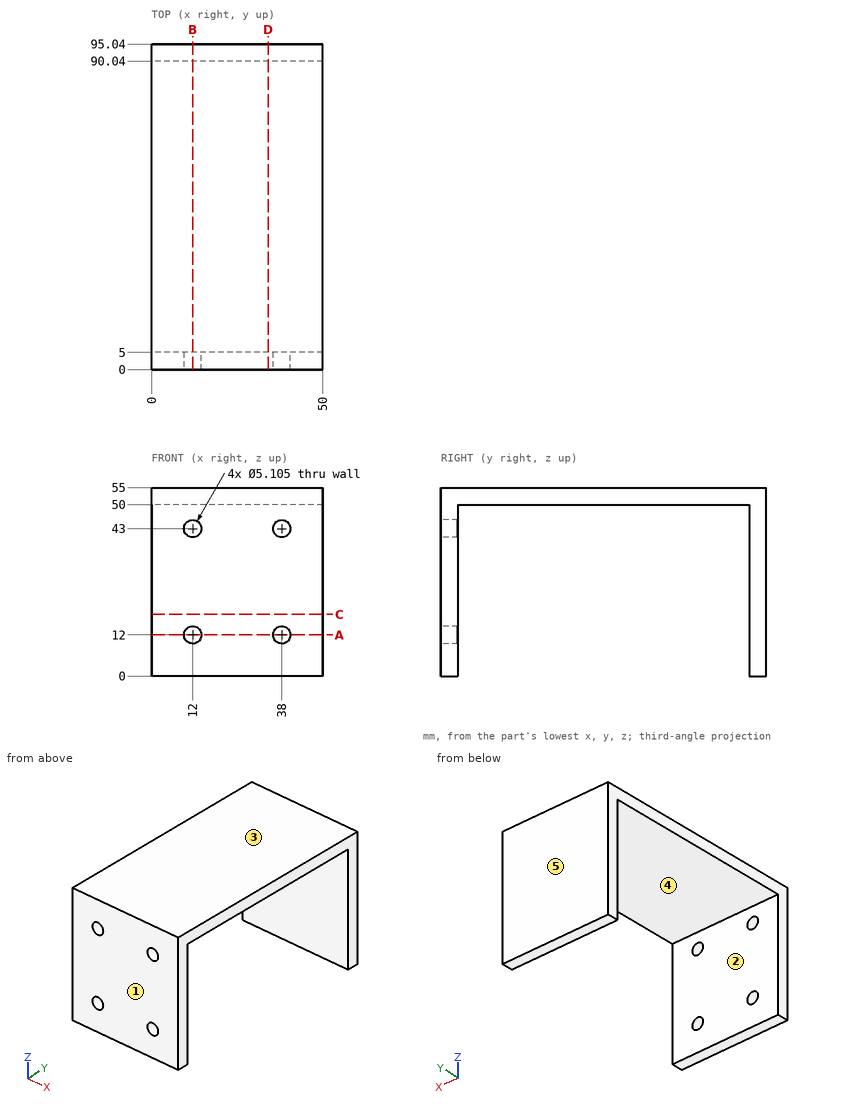
Input: dimensioned drawing with shaded views. Units: mm. Origin: part minimum x, y, z. A direction names the side the tool comes from. Round coordinates to 2 decimals unless told otherwise and drop trailing zeros. Order: outer loops, then holes, each group sorted by start corner. A loop starts at its lowest first (then second) coordinate and runs counter-clockwise, first axis right, second up. Notation, with made-up numbers: M 35,-17.5 L 48,-17.5 A10 ccw 48,-11.5 Z; hole C -26.5,-38 d11. An arc over 180 degrees is marked long. Use one line per item in the form item = value. Start each with the question number.
Q1. Cut plane A-A (z = 12). Return loops of the section in (x, y).
Q2. Access query for the marked faces 1 and 2. Directions: +Z, -Z, +X, -X, +Y, -Y. A direction counts if a zero-diameter tool reaches every point of the face in a straight line with its end or side. Return the directions, or none.
Q3. Cut plane B-B (x = 12). Return loops of the section in (y, z), and give its area (3 significant figures).
Q4. Pin query (flat end, axial travel): pin 1 Ø10 at (x, y) = (36.5, 48) entering from -Z. Return the tip coordinate at first contact, or that it passes through.
Q5. Mould query, pull axis Y, two halves, no side actions, for the marked faces 3, 4 and 5. Classes: +Y half, -Y half, draft (parallel to the pull), parting line (faces both ways), or undercut.
Q6. Cut plane C-C (z = 18). Return loops of the section in (x, y).
Q7. Cut plane D-D (x = 34). Return loops of the section in (y, z).
Q8. Material intervals for line 1 (Z direction, x = 12, y = 2); line 2 (X direction, y = 3.15, z = 12); line 3 (Y direction, x = 9.5, z = 28), sorted ascending. Write a range as [from, to].
Geometry results:
q1.outline = M 0,0 L 9.45,0 L 9.45,5 L 0,5 Z; M 0,90.04 L 50,90.04 L 50,95.04 L 0,95.04 Z; M 14.55,0 L 35.45,0 L 35.45,5 L 14.55,5 Z; M 40.55,0 L 50,0 L 50,5 L 40.55,5 Z
q2.face_1 = +Z, -Z, +X, -X, -Y
q2.face_2 = -Z, +X, -X
q3.outline = M 0,0 L 5,0 L 5,9.45 L 0,9.45 Z; M 0,14.55 L 5,14.55 L 5,40.45 L 0,40.45 Z; M 0,45.55 L 5,45.55 L 5,50 L 90.04,50 L 90.04,0 L 95.04,0 L 95.04,55 L 0,55 Z
q3.area = 924 mm^2
q4.pin_1 = 50
q5.face_3 = draft
q5.face_4 = undercut
q5.face_5 = +Y half
q6.outline = M 0,0 L 50,0 L 50,5 L 0,5 Z; M 0,90.04 L 50,90.04 L 50,95.04 L 0,95.04 Z
q7.outline = M 0,0 L 5,0 L 5,50 L 90.04,50 L 90.04,0 L 95.04,0 L 95.04,55 L 0,55 Z
q8.line_1 = [0, 9.45], [14.55, 40.45], [45.55, 55]
q8.line_2 = [0, 9.45], [14.55, 35.45], [40.55, 50]
q8.line_3 = [0, 5], [90.04, 95.04]
